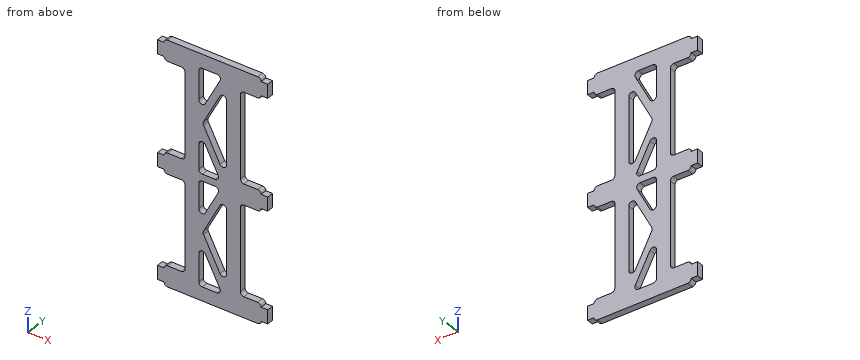
from build123d import *

# Parameters (mm, degrees)
SKETCH1_W           = 25.4
SKETCH1_H           = 111.125
BOSS_EXTRUDE1_DEPTH = 1.5
SKETCH2_W           = 9.525
SKETCH2_H           = 9.525
BOSS_EXTRUDE2_DEPTH = 3
CUT_EXTRUDE1_DEPTH  = 178.633881287
FILLET1_R           = 1.5875
SKETCH5_W           = 3
SKETCH5_H           = 6.35
BOSS_EXTRUDE3_DEPTH = 3


with BuildPart() as part:
    # Sketch1 → Boss-Extrude1 (new, symmetric)
    with BuildSketch(Plane(origin=(0, 34.29, 0), x_dir=(1, 0, 0), z_dir=(0, 1, 0))):
        with Locations((0, 120.65)):
            Rectangle(SKETCH1_W, SKETCH1_H)
    extrude(amount=BOSS_EXTRUDE1_DEPTH, both=True)

    # Sketch2 → Boss-Extrude2 (add)
    with BuildSketch(Plane(origin=(0, 35.79, 0), x_dir=(1, 0, 0), z_dir=(0, 1, 0))):
        with Locations((17.4625, 171.45)):
            Rectangle(SKETCH2_W, SKETCH2_H)
        with Locations((-17.4625, 171.45)):
            Rectangle(SKETCH2_W, SKETCH2_H)
        with Locations((17.4625, 120.65)):
            Rectangle(SKETCH2_W, SKETCH2_H)
        with Locations((-17.4625, 120.65)):
            Rectangle(SKETCH2_W, SKETCH2_H)
        with Locations((17.4625, 69.85)):
            Rectangle(SKETCH2_W, SKETCH2_H)
        with Locations((-17.4625, 69.85)):
            Rectangle(SKETCH2_W, SKETCH2_H)
    extrude(amount=-BOSS_EXTRUDE2_DEPTH)

    # Sketch4 → Cut-Extrude1 (cut, through all)
    with BuildSketch(Plane(origin=(0, 35.79, 0), x_dir=(1, 0, 0), z_dir=(0, 1, 0))):
        Polygon((4.563523411, 71.4375), (-6.35, 92.58245161), (-6.35, 71.4375), align=None)
        Polygon((6.35, 74.89879839), (6.35, 117.18870161), (-4.563523411, 96.04375), align=None)
        Polygon((3.744168573, 119.0625), (-6.35, 119.0625), (-6.35, 99.50504839), align=None)
        Polygon((3.744168573, 122.2375), (-6.35, 141.79495161), (-6.35, 122.2375), align=None)
        Polygon((6.35, 124.11129839), (6.35, 166.40120161), (-4.563523411, 145.25625), align=None)
        Polygon((4.563523411, 169.8625), (-6.35, 169.8625), (-6.35, 148.71754839), align=None)
    extrude(amount=-CUT_EXTRUDE1_DEPTH, mode=Mode.SUBTRACT)

    # Fillet1
    fillet1_edges = [part.edges().sort_by_distance(p)[0] for p in [
        (3.744168573, 34.29, -119.0625),
        (-6.35, 34.29, -99.50504839),
        (-6.35, 34.29, -119.0625),
        (-4.563523411, 34.29, -96.04375),
        (6.35, 34.29, -117.18870161),
        (6.35, 34.29, -74.89879839),
        (-4.563523411, 34.29, -145.25625),
        (6.35, 34.29, -166.40120161),
        (6.35, 34.29, -124.11129839),
        (3.744168573, 34.29, -122.2375),
        (-6.35, 34.29, -122.2375),
        (-6.35, 34.29, -141.79495161),
        (-6.35, 34.29, -148.71754839),
        (-6.35, 34.29, -169.8625),
        (4.563523411, 34.29, -169.8625),
        (4.563523411, 34.29, -71.4375),
        (-6.35, 34.29, -71.4375),
        (-6.35, 34.29, -92.58245161),
        (22.225, 34.29, -65.0875),
        (22.225, 34.29, -74.6125),
        (12.7, 34.29, -74.6125),
        (-12.7, 34.29, -115.8875),
        (-12.7, 34.29, -125.4125),
        (-22.225, 34.29, -125.4125),
        (-22.225, 34.29, -115.8875),
        (22.225, 34.29, -115.8875),
        (22.225, 34.29, -125.4125),
        (12.7, 34.29, -125.4125),
        (12.7, 34.29, -115.8875),
        (-12.7, 34.29, -166.6875),
        (-22.225, 34.29, -176.2125),
        (-22.225, 34.29, -166.6875),
        (-12.7, 34.29, -74.6125),
        (-22.225, 34.29, -74.6125),
        (-22.225, 34.29, -65.0875),
        (22.225, 34.29, -166.6875),
        (22.225, 34.29, -176.2125),
        (12.7, 34.29, -166.6875),
    ]]
    fillet(fillet1_edges, radius=FILLET1_R)

    # Sketch5 → Boss-Extrude3 (add)
    with BuildSketch(Plane(origin=(0, 35.79, 0), x_dir=(1, 0, 0), z_dir=(0, 1, 0))):
        with Locations((23.725, 171.45)):
            Rectangle(SKETCH5_W, SKETCH5_H)
        with Locations((-23.725, 171.45)):
            Rectangle(SKETCH5_W, SKETCH5_H)
        with Locations((23.725, 120.65)):
            Rectangle(SKETCH5_W, SKETCH5_H)
        with Locations((-23.725, 120.65)):
            Rectangle(SKETCH5_W, SKETCH5_H)
        with Locations((23.725, 69.85)):
            Rectangle(SKETCH5_W, SKETCH5_H)
        with Locations((-23.725, 69.85)):
            Rectangle(SKETCH5_W, SKETCH5_H)
    extrude(amount=-BOSS_EXTRUDE3_DEPTH)


solid = part.part
Geometry: final body of the model. Coordinates: model frame, mm. Coordinates: 2 decimals unless noted, no trailing zeros. Write each loop counter-clockwise with the first axis right and the second up, starting at its lowest first coordinate (ties: lowest second). Pieces come first, ordered by that corner, then holes. Notation, with made-up numbers: (47, 34.25) - (66, 34.25) arc R30 cw to (66, 73.25) - close; hole circle Ø7 at (-33, 4). An arc over 180 degrees is marked (long way). Return JSON: item names as keys, results as strings.
Item 1: Section query C-C (y = 34.6). Count the separate pieces of the cut face and the enclosed holes in it, and give its area (3 significant figures).
Completed:
{"separate pieces": "1", "enclosed holes": "6", "area": "2,650 mm2"}
Item 2: Section query A-A (x = 19.5). Output: boundary loops of the cut face in (y, z), and give its area (3 significant figures).
Completed:
{"outline": "(32.79, -176.21) - (35.79, -176.21) - (35.79, -166.69) - (32.79, -166.69) - close; (32.79, -125.41) - (35.79, -125.41) - (35.79, -115.89) - (32.79, -115.89) - close; (32.79, -74.61) - (35.79, -74.61) - (35.79, -65.09) - (32.79, -65.09) - close", "area": "85.7 mm2"}
Item 3: Section query B-B (z = -108.5). Output: boundary loops of the cut face in (x, y).
Completed:
{"outline": "(-12.7, 32.79) - (-6.35, 32.79) - (-6.35, 35.79) - (-12.7, 35.79) - close; (-1.71, 32.79) - (1.87, 32.79) - (1.87, 35.79) - (-1.71, 35.79) - close; (6.35, 32.79) - (12.7, 32.79) - (12.7, 35.79) - (6.35, 35.79) - close"}
Item 4: Pin query (flat end, axial travel): pin 1 Ø0.9 at (x, y) = (-23.5, 34.5) entering from +Z (3 decimals); pin 2 Ø0.9 at (x, y) = (23.5, 35) entering from -Z (3 decimals); pin 3 Ø1.5 at (y, z) = (34.5, -148.5) entering from -X. Return the tip coordinate at first contact, or that it passes through.
Completed:
{"pin 1": "stops at z = -66.675", "pin 2": "stops at z = -174.625", "pin 3": "stops at x = -12.7"}
Item 5: Line query: L1, parallel to Z at x = 19.5, y = 34.8; L2, parallel to X at y = 35.45, z = -82; L3, parallel to X at y = 34.05, z = -81. Output: solid intervals per line, ascending.
Completed:
{"L1": "z = -176.21 to -166.69, -125.41 to -115.89, -74.61 to -65.09", "L2": "x = -12.7 to -6.35, -0.89 to 2.68, 6.35 to 12.7", "L3": "x = -12.7 to -6.35, -0.37 to 3.2, 6.29 to 12.7"}
